Design review of the part built by this model. Coordinates are the model's own, in mm. Give positions to 0.01 mm unless a question says otherwise; leave off trailing zeros. Write each loop counter-clockwise with the first axis right and the second up, starting at its lowest first coordinate (ties: lowest second). Pieces come first, ordered by that corner, then holes. Notation, with made-up numbers: (-12.75, 47) -> (34.25, 47) arc R31 cw to (34.25, 78) -> close; hole circle Ø10 at (25, 66). An arc over 180 degrees is marked (long way). Use CSV: the item, a comma, the result in double quotes.
```python
from build123d import *

# Parameters (mm, degrees)
SKETCH1_R           = 15
SKETCH1_R_2         = 4
BOSS_EXTRUDE1_DEPTH = 3
SKETCH2_R           = 4
SKETCH2_R_2         = 3.5
BOSS_EXTRUDE2_DEPTH = 5
SKETCH4_R           = 4
BOSS_EXTRUDE4_DEPTH = 3


with BuildPart() as part:
    # Sketch1 → Boss-Extrude1 (new body)
    with BuildSketch(Plane.XY):
        with Locations((-0.860205172, 39.990749519)):
            Circle(SKETCH1_R)
        with Locations((-0.860205172, 39.990749519)):
            Circle(SKETCH1_R_2, mode=Mode.SUBTRACT)
    extrude(amount=BOSS_EXTRUDE1_DEPTH)



with BuildPart() as body_2:
    # Sketch2 → Boss-Extrude2 (new body)
    with BuildSketch(Plane(origin=(0, 0, 0), x_dir=(-1, 0, 0), z_dir=(0, 0, -1))):
        with Locations(Location((0.860205172, 39.990749519, 0), (0, 0, 180))):
            Circle(SKETCH2_R)
        with Locations((0.860205172, 39.990749519)):
            Circle(SKETCH2_R_2, mode=Mode.SUBTRACT)
    extrude(amount=BOSS_EXTRUDE2_DEPTH)


with BuildPart() as part_1:
    add(part.part)

    add(body_2.part)  # Boss-Extrude4 merges body 2
    # Sketch4 → Boss-Extrude4 (add)
    with BuildSketch(Plane.XY):
        with Locations((-0.860205172, 39.990749519)):
            Circle(SKETCH4_R)
    extrude(amount=BOSS_EXTRUDE4_DEPTH)


solid = part_1.part
```
(1) Mouldability with a two-part tool opening along Y and no side actions: class faces 1 (the face through (-2.813, 54.863, 1.479)), 2 (the face through (-1, 40, 0)), 3 (the face through (-1, 40, 3)) as +Y half, -Y half, draft (parallel to the pull), parting line (faces both ways), or undercut.
Established:
face 1,"parting line"
face 2,"undercut"
face 3,"draft"
(2) For line 1 along X through (y, z) = (40, -4); line 2 along Z through (x, y) = (9.5, 42.25); line 3 along Y through (x, z) = (1, -1.25), list the stretches that pass through material, from the lowest coordinate up. Write a range as [from, to].
Established:
line 1,"x = [-4.86, -4.36], [2.64, 3.14]"
line 2,"z = [0, 3]"
line 3,"y = [36.45, 37.03], [42.96, 43.53]"
(3) Take a section at D-D (z = 1.75). Write out the cut boundary in (x, y).
Established:
outline,"circle Ø30 at (-0.86, 39.99)"
(4) Clearance check with flat-ended pins moving along their axes: pin 1 (2 mm diameter, centred on x = -9.5, y = 50, fed in from -Z); pin 2 (4 mm diameter, centred on y = 29.5, z = -3.5, fed in from +X); pin 3 (3 mm diameter, centred on x = 7, z = 0, fed in from +Y). State where each tip first meets the part, or that it passes through.
Established:
pin 1,"stops at z = 0"
pin 2,"passes through"
pin 3,"stops at y = 53.58"
(5) Take a section at A-A (x = -3.75). Write out the cut boundary in (y, z).
Established:
outline,"(25.27, 0) -> (37.23, 0) -> (37.23, -5) -> (38.02, -5) -> (38.02, 0) -> (41.97, 0) -> (41.97, -5) -> (42.76, -5) -> (42.76, 0) -> (54.71, 0) -> (54.71, 3) -> (25.27, 3) -> close"
(6) Take a section at C-C (z = -3.5). Write out the cut boundary in (x, y).
Established:
outline,"circle Ø8 at (-0.86, 39.99); hole circle Ø7 at (-0.86, 39.99)"
(7) Take a section at B-B (y = 49). Write out the cut boundary in (x, z).
Established:
outline,"(-12.85, 0) -> (11.13, 0) -> (11.13, 3) -> (-12.85, 3) -> close"
